The model under review builds one solid part; all positions refer to its coordinate system, in mm. Face numbers are marked on the shaded views. A direction names the side the tool comes from. Round coordinates to 2 decimals unless told otherwise and drop trailing zeros. Order: outer loops, then holes, each group sorted by start corner. A loop starts at its lowest first (then second) coordinate and runs counter-clockwise, first axis right, second up. Notation, with made-up numbers: M 54,32 L 105,32 A35 cw 105,67 Z; hole C 79.5,56 d10. An arc over 180 degrees is marked long. Answer as a JSON object with one key per item and string values. Group by question number.
1. Clearance check with flat-ended pins moving along their axes: P1, Ø1.5, axis at x = 5.5, y = 2, coming from the -Z side; P2, Ø1.6, axis at x = 0.5, z = 1, coming from the +Y side; P3, Ø1.9, axis at x = 0, z = 6.735, coming from the -Y side; P4, Ø1, axis at x = 2.5, y = 1, coming from the +Z side. State where each tip first meets the part, or that it passes through.
2. To check wall thickness, follow probe 1 along Y at (x, z) = (-1.5, -5.75); probe 2 along X at (y, z) = (3.5, 2.25); probe 3 along X at (y, z) = (2.4, 0.25). State the ranges of each line that lie inside material, in increasing order. Write a range as [from, to].
3. Mouldability with a two-part tool opening along Z and no side actions: class the marked faces 1, 2 and 3 as released by +Z, released by -Z, zero draft, split by the parting line, or undercut.
4. Add section C-C on x = 7.5. State the section outline as (y, z) points, and give its area (3 significant figures).
5. Add section A-A on x = 0. State the section outline as (y, z) points (3 decimals).
6. Add section D-D on z = 7.5. State the section outline as (x, y) points.
7. Add section B-B on z = 0. State the section outline as (x, y) points (3 decimals), and give its area (3 significant figures).
8. Machinability: for the marked faces 4 and 5, which of the approach directions +Z, -Z, +X, -X, +Y, -Y give a long, thin tool a straight path to every point of the face, cutting with its end or side? Answer none if there is none.
```python
from build123d import *

# Parameters (mm, degrees)
SKETCH1_R           = 10
BOSS_EXTRUDE1_DEPTH = 2.05
SKETCH2_R           = 4.75
BOSS_EXTRUDE2_DEPTH = 3.5
SKETCH3_R           = 2.725
CUT_EXTRUDE1_DEPTH  = 3.55
SKETCH4_R           = 1.375
CUT_EXTRUDE2_DEPTH  = 3.55
SKETCH5_R           = 1.205
CUT_EXTRUDE3_DEPTH  = 3.55
CIRPATTERN1_COUNT   = 4


with BuildPart() as part:
    # Sketch1 → Boss-Extrude1 (new body)
    with BuildSketch(Plane(origin=(0, 0, 0), x_dir=(1, 0, 0), z_dir=(0, 1, 0))):
        Circle(SKETCH1_R)
    extrude(amount=BOSS_EXTRUDE1_DEPTH)

    # Sketch2 → Boss-Extrude2 (add)
    with BuildSketch(Plane(origin=(0, 2.05, 0), x_dir=(1, 0, 0), z_dir=(0, 1, 0))):
        Circle(SKETCH2_R)
    extrude(amount=BOSS_EXTRUDE2_DEPTH)

    # Sketch3 → Cut-Extrude1 (cut)
    with BuildSketch(Plane(origin=(0, 5.55, 0), x_dir=(1, 0, 0), z_dir=(0, 1, 0))):
        Circle(SKETCH3_R)
    extrude(amount=-CUT_EXTRUDE1_DEPTH, mode=Mode.SUBTRACT)

    # Sketch4 → Cut-Extrude2 (cut)
    with BuildSketch(Plane(origin=(0, 2, 0), x_dir=(1, 0, 0), z_dir=(0, 1, 0))):
        Circle(SKETCH4_R)
    extrude(amount=-CUT_EXTRUDE2_DEPTH, mode=Mode.SUBTRACT)

    # Sketch5 → Cut-Extrude3 (cut)
    with BuildSketch(Plane.XZ):
        with Locations((-6.735, 0)):
            Circle(SKETCH5_R)
    cut_extrude3 = extrude(amount=-CUT_EXTRUDE3_DEPTH, mode=Mode.SUBTRACT)

    # CirPattern1: Cut-Extrude3 ×4 about axis
    cirpattern1_axis = Axis((0, 0, 0), (0, 1, 0))
    for i in range(1, CIRPATTERN1_COUNT):
        add(cut_extrude3.rotate(cirpattern1_axis, i * 360 / CIRPATTERN1_COUNT), mode=Mode.SUBTRACT)


solid = part.part
```
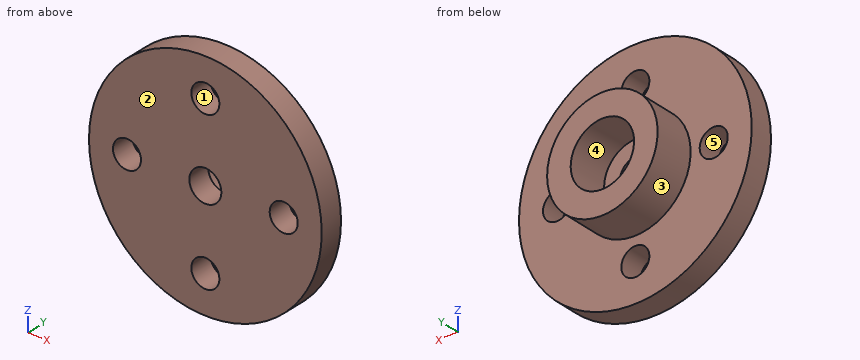
Recorded:
{
 "1": {"P1": "stops at z = -8.8", "P2": "stops at y = 2", "P3": "passes through", "P4": "stops at z = 9.8"},
 "2": {"probe 1": "y = [0, 2.05]", "probe 2": "x = [-4.18, -1.54], [1.54, 4.18]", "probe 3": "x = [-4.74, -2.71], [2.71, 4.74]"},
 "3": {"face 1": "undercut", "face 2": "zero draft", "face 3": "split by the parting line"},
 "4": {"outline": "M 0,-6.61 L 2.05,-6.61 L 2.05,-0.93 L 0,-0.93 Z; M 0,0.93 L 2.05,0.93 L 2.05,6.61 L 0,6.61 Z", "area": "23.3 mm²"},
 "5": {"outline": "M 0,-10 L 2.05,-10 L 2.05,-7.94 L 0,-7.94 Z; M 0,-5.53 L 2.05,-5.53 L 2.05,-4.75 L 5.55,-4.75 L 5.55,-2.725 L 2,-2.725 L 2,-1.375 L 0,-1.375 Z; M 0,1.375 L 2,1.375 L 2,2.725 L 5.55,2.725 L 5.55,4.75 L 2.05,4.75 L 2.05,5.53 L 0,5.53 Z; M 0,7.94 L 2.05,7.94 L 2.05,10 L 0,10 Z"},
 "6": {"outline": "M -6.61,0 L -0.93,0 L -0.93,2.05 L -6.61,2.05 Z; M 0.93,0 L 6.61,0 L 6.61,2.05 L 0.93,2.05 Z"},
 "7": {"outline": "M -10,0 L -7.94,0 L -7.94,2.05 L -10,2.05 Z; M -5.53,0 L -1.375,0 L -1.375,2 L -2.725,2 L -2.725,5.55 L -4.75,5.55 L -4.75,2.05 L -5.53,2.05 Z; M 1.375,0 L 5.53,0 L 5.53,2.05 L 4.75,2.05 L 4.75,5.55 L 2.725,5.55 L 2.725,2 L 1.375,2 Z; M 7.94,0 L 10,0 L 10,2.05 L 7.94,2.05 Z", "area": "39.5 mm²"},
 "8": {"face 4": "+Y", "face 5": "+Y, -Y"}
}
